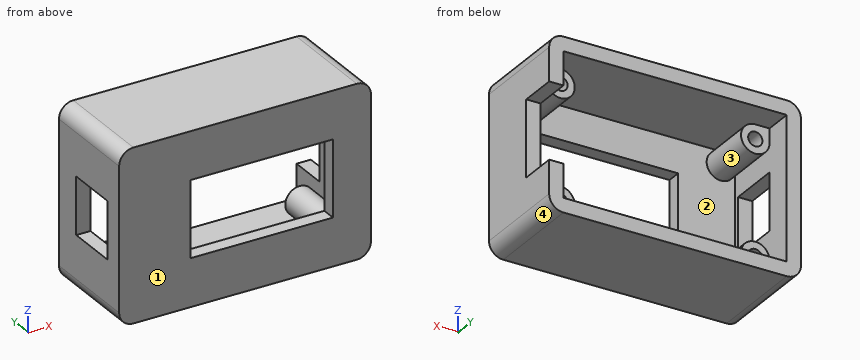
Autodesk Fusion 360 part; units mm, degrees
sketch "Sketch1" plane through (0, 0, 0) normal (0, 1, 0) x (1, 0, 0)
  line L0 (0, 0) -> (53, 0)
  line L1 (53, 0) -> (53, -36)
  line L2 (53, -36) -> (0, -36)
  line L3 (0, -36) -> (0, 0)
extrude "Extrude1" add sketch "Sketch1" along normal blind 3
sketch "Sketch2" plane through (0, 3, 0) normal (0, 1, 0) x (-1, 0, 0)
  line L0 (0, 36) -> (-53, 36)
  line L1 (-53, 36) -> (-53, 0)
  line L2 (-53, 0) -> (0, 0)
  line L3 (0, 0) -> (0, 36)
  line L4 (-3, 3) -> (-50, 3)
  line L5 (-50, 3) -> (-50, 33)
  line L6 (-50, 33) -> (-3, 33)
  line L7 (-3, 33) -> (-3, 3)
  circle A0 centre (-47, 30) radius 3
  circle A1 centre (-47, 6) radius 3
  circle A2 centre (-6, 30) radius 3
  circle A3 centre (-6, 6) radius 3
  circle A4 centre (-6, 6) radius 1.5
  circle A5 centre (-6, 30) radius 1.5
  circle A6 centre (-47, 30) radius 1.5
  circle A7 centre (-47, 6) radius 1.5
  dimension "d3" = 6
  dimension "d4" = 6
  dimension "d5" = 3
  dimension "d6" = 3
  dimension "d7" = 3
extrude "Extrude2" add sketch "Sketch2" along normal blind 12 contours L4 L7 A3 | A3 | L4 L5 A1 | A1 | L6 L7 A2 | A2 | L5 L6 A0 | A0
extrude "Extrude3" add sketch "Sketch2" along normal blind 18 contours L0 L1 L2 L3
sketch "Sketch3" plane through (0, 0, 0) normal (-1, 0, 0) x (0, 0, 1)
  line L0 (0, 0) -> (36, 0)
  line L1 (36, 0) -> (36, 21)
  line L2 (36, 21) -> (0, 21)
  line L3 (0, 21) -> (0, 0)
  line L4 (12.0161, 21) -> (24.0161, 21)
  line L5 (24.0161, 21) -> (24.0161, 4)
  line L6 (24.0161, 4) -> (12.0161, 4)
  line L7 (12.0161, 4) -> (12.0161, 21)
  line L8 (12.0161, 21) -> (24.0161, 21)
  line L9 (24.0161, 21) -> (24.0161, 15)
  line L10 (24.0161, 15) -> (12.0161, 15)
  line L11 (12.0161, 15) -> (12.0161, 21)
  dimension "d12" = 12
  dimension "d13" = 17
  dimension "d14" = 6
extrude "Extrude4" cut sketch "Sketch3" against normal blind 11 contours L5 L6 L7 L10
sketch "Sketch4" plane through (53, 0, 0) normal (1, 0, 0) x (0, 0, -1)
  line L0 (-36, 0) -> (0, 0)
  line L1 (0, 0) -> (0, 21)
  line L2 (0, 21) -> (-36, 21)
  line L3 (-36, 21) -> (-36, 0)
  line L4 (-9.9926, 21) -> (-25.9926, 21)
  line L5 (-25.9926, 21) -> (-25.9926, 13)
  line L6 (-25.9926, 13) -> (-9.9926, 13)
  line L7 (-9.9926, 13) -> (-9.9926, 21)
  dimension "d17" = 16
extrude "Extrude5" cut sketch "Sketch4" against normal blind 6 contours L2 L4 L5 L6 L7
fillet "Fillet1" radius 3 1 edges at (53, 10.5, 0)
fillet "Fillet2" radius 3 1 edges at (0, 10.5, 0)
fillet "Fillet3" radius 3 1 edges at (0, 10.5, 36)
fillet "Fillet4" radius 3 1 edges at (53, 10.5, 36)
sketch "Sketch5" plane through (0, 0, 0) normal (0, -1, 0) x (1, 0, 0)
  arc A0 (53, 33) -> (50, 36) centre (50, 33) ccw
  line L0 (50, 36) -> (3, 36)
  arc A1 (3, 36) -> (0, 33) centre (3, 33) ccw
  line L1 (0, 33) -> (0, 3)
  arc A2 (0, 3) -> (3, 0) centre (3, 3) ccw
  line L2 (3, 0) -> (50, 0)
  arc A3 (50, 0) -> (53, 3) centre (50, 3) ccw
  line L3 (53, 3) -> (53, 33)
  line L4 (50, 10.0095) -> (15, 10.0095)
  line L5 (15, 10.0095) -> (15, 26.0095)
  line L6 (15, 26.0095) -> (50, 26.0095)
  line L7 (50, 26.0095) -> (50, 10.0095)
  line L8 (50, 10.0095) -> (45, 10.0095)
  line L9 (45, 10.0095) -> (45, 26.0095)
  line L10 (45, 26.0095) -> (50, 26.0095)
  line L11 (50, 26.0095) -> (50, 10.0095)
  dimension "d28" = 16
  dimension "d29" = 5
extrude "Extrude6" cut sketch "Sketch5" against normal blind 7 contours L4 L5 L6 L9
Read the model definition and answer for the solid it produces. Units are mm, in the model's axes. Face numbers are marked on the shaded views. Coordinates: 2 decimals unless noted, no trailing zeros. Write each loop counter-clockwise with the first axis right and the second up, starting at its lowest first coordinate (ties: lowest second). Pieces come first, ordered by that corner, then holes. Notation, with made-up numbers: (25.25, 46) -> (58.25, 46) arc R23 cw to (58.25, 71) -> close; hole circle Ø2 at (-7.5, -3.5). An arc over 180 degrees is marked (long way). Answer as a JSON object with one key per item and string values.
Q1. The part is cut by section C-C on y = 12.25. Give the vertices of the cut face in (x, z), then the cut area to 3 significant figures.
The answers:
{"outline": "(0, 3) arc R3 ccw to (3, 0) -> (50, 0) arc R3 ccw to (53, 3) -> (53, 33) arc R3 ccw to (50, 36) -> (3, 36) arc R3 ccw to (0, 33) -> (0, 24.02) -> (3, 24.02) -> (3, 30) arc R3 ccw (long way) to (6, 33) -> (47, 33) arc R3 ccw (long way) to (50, 30) -> (50, 6) arc R3 ccw (long way) to (47, 3) -> (6, 3) arc R3 ccw (long way) to (3, 6) -> (3, 12.02) -> (0, 12.02) -> close; hole circle Ø3 at (6, 6); hole circle Ø3 at (6, 30); hole circle Ø3 at (47, 6); hole circle Ø3 at (47, 30)", "area": "547 mm2"}
Q2. Flat-ended cylindrical pins translate along their axes: pin 1 Ø6.5 at (x, z) = (48, 7.5) entering from +Y; pin 2 Ø1.5 at (x, z) = (51.5, 19) entering from +Y; pin 3 Ø2.5 at (x, z) = (6, 30) entering from +Y. Find the tip coordinate at first contact, or state that the pin passes through.
The answers:
{"pin 1": "stops at y = 21", "pin 2": "stops at y = 13", "pin 3": "stops at y = 3"}
Q3. The part is cut by section D-D on x = 14. Give the vertices of the cut face in (y, z), then the cut area to 3 significant figures.
The answers:
{"outline": "(0, 0) -> (21, 0) -> (21, 3) -> (3, 3) -> (3, 33) -> (21, 33) -> (21, 36) -> (0, 36) -> close", "area": "216 mm2"}
Q4. Determine the mould class of the marked faces 1, 2, 3 and 4 for opening direction Z: pulls with the +Z half, pulls with the -Z half, needs draft (parallel to the pull), parting line crosses it, or undercut.
The answers:
{"face 1": "needs draft", "face 2": "undercut", "face 3": "undercut", "face 4": "pulls with the -Z half"}
Q5. The part is cut by section B-B on z = 25. Give the vertices of the cut face in (x, y).
The answers:
{"outline": "(0, 0) -> (15, 0) -> (15, 3) -> (3, 3) -> (3, 21) -> (0, 21) -> close; (45, 0) -> (53, 0) -> (53, 13) -> (50, 13) -> (50, 3) -> (45, 3) -> close"}
Q6. Consider line 1 (Z direction, x = 28, y = 12.75); line 2 (X direction, y = 18.5, z = 31); line 3 (X direction, y = 1.5, z = 11). Determine where each line is inside the solid, lowest interval first. Write a range as [from, to].
The answers:
{"line 1": "z = [0, 3], [33, 36]", "line 2": "x = [0, 3], [50, 53]", "line 3": "x = [0, 15], [45, 53]"}
Q7. The part is cut by section A-A on x = 36.5. Give the vertices of the cut face in (y, z), then the cut area to 3 significant figures.
The answers:
{"outline": "(0, 0) -> (21, 0) -> (21, 3) -> (3, 3) -> (3, 10.01) -> (0, 10.01) -> close; (0, 26.01) -> (3, 26.01) -> (3, 33) -> (21, 33) -> (21, 36) -> (0, 36) -> close", "area": "168 mm2"}
